Build history of the part. All positions in model axes, mm. Give positions to 0.01 mm unless a question says otherwise; leave off trailing zeros. Write each loop counter-clockwise with the first axis right and the second up, starting at its lowest first coordinate (ties: lowest second). Pieces come first, ordered by that corner, then holes. Notation, with made-up numbers: (-4.75, 31.5) -> (33.25, 31.5) arc R24 cw to (33.25, 48.5) -> close; hole circle Ø7 at (-27, 34). An arc over 180 degrees is marked (long way). Write item = value, one per line. Start each with the question number.
Q1. Mould opens along Z. For faces 1 (the face through (0, 0, 6.747)), 2 (the face through (0, 0, -6.747)), 3 (the face through (0.93, 0.21, 5.97)) say: pulls with the +Z half, pulls with the -Z half, needs draft (parallel to the pull), parting line crosses it, or undercut.
Q2. Saw through at C-C, the plane z = -3. List the corners of the cut face in (x, y), then the cut area to 3 significant figures.
Q3. Saw through at A-A, the plane y = 0. List the corners of the cut face in (x, z), then the cut area to 3 significant figures.
Q4. Wall check: line 1 (Z direction, x = -0.25, y = 1); line 2 (Y direction, x = -0.1, z = -3); line 3 (Y direction, x = -0.85, z = 3). Give the ranges that are in metal, low to high.
from build123d import *

# Parameters (mm, degrees)
SKETCH1_R           = 1.49987
BOSS_EXTRUDE1_DEPTH = 6.746875
SKETCH2_W           = 0.54
SKETCH2_H           = 0.54737
CHAMFER1_SIZE       = 0.254


with BuildPart() as part:
    # Sketch1 → Boss-Extrude1 (new body, symmetric)
    with BuildSketch(Plane.XY):
        Circle(SKETCH1_R)
    extrude(amount=BOSS_EXTRUDE1_DEPTH, both=True)

    # Sketch2 → Cut-Revolve1 (revolve, cut)
    with BuildSketch(Plane(origin=(0, 0, 0), x_dir=(0, 0, -1), z_dir=(1, 0, 0))):
        with Locations((-5.968875, -1.226185)):
            Rectangle(SKETCH2_W, SKETCH2_H)
    revolve(axis=Axis((0, 0, 8.828032455), (0, 0, -1)), mode=Mode.SUBTRACT)

    # Chamfer1
    chamfer1_edges = [part.edges().sort_by_distance(p)[0] for p in [
        (-1.49987, 0, -6.746875),
        (-1.49987, 0, 6.746875),
    ]]
    chamfer(chamfer1_edges, length=CHAMFER1_SIZE)


solid = part.part
Report:
q1.face_1 = pulls with the +Z half
q1.face_2 = pulls with the -Z half
q1.face_3 = undercut
q2.outline = circle Ø3 at (0, 0)
q2.area = 7.07 mm2
q3.outline = (-1.5, -6.49) -> (-1.25, -6.75) -> (1.25, -6.75) -> (1.5, -6.49) -> (1.5, 5.7) -> (0.95, 5.7) -> (0.95, 6.24) -> (1.5, 6.24) -> (1.5, 6.49) -> (1.25, 6.75) -> (-1.25, 6.75) -> (-1.5, 6.49) -> (-1.5, 6.24) -> (-0.95, 6.24) -> (-0.95, 5.7) -> (-1.5, 5.7) -> close
q3.area = 39.8 mm2
q4.line_1 = -6.75 to 5.7, 6.24 to 6.75
q4.line_2 = -1.5 to 1.5
q4.line_3 = -1.24 to 1.24
